Answer from the drawing. Dimensions are ordinates in mm from the lowest x, y and z of the part. A direction names the side the tool comes from. Round coordinates to 2 decimals unless told otherwise and drop trailing zeros. Loops run counter-clockwise (first coordinate to the right, second up) from the corner with the lowest first, then second, coordinate; pieces in that order, holes last. Notation, with made-up numbers: M -29.5,42.25 L -22.5,42.25 A26 cw -22.5,69.25 Z; hole C -15,2 d6. An arc over 180 degrees is marked long. One line per item, written item: value.
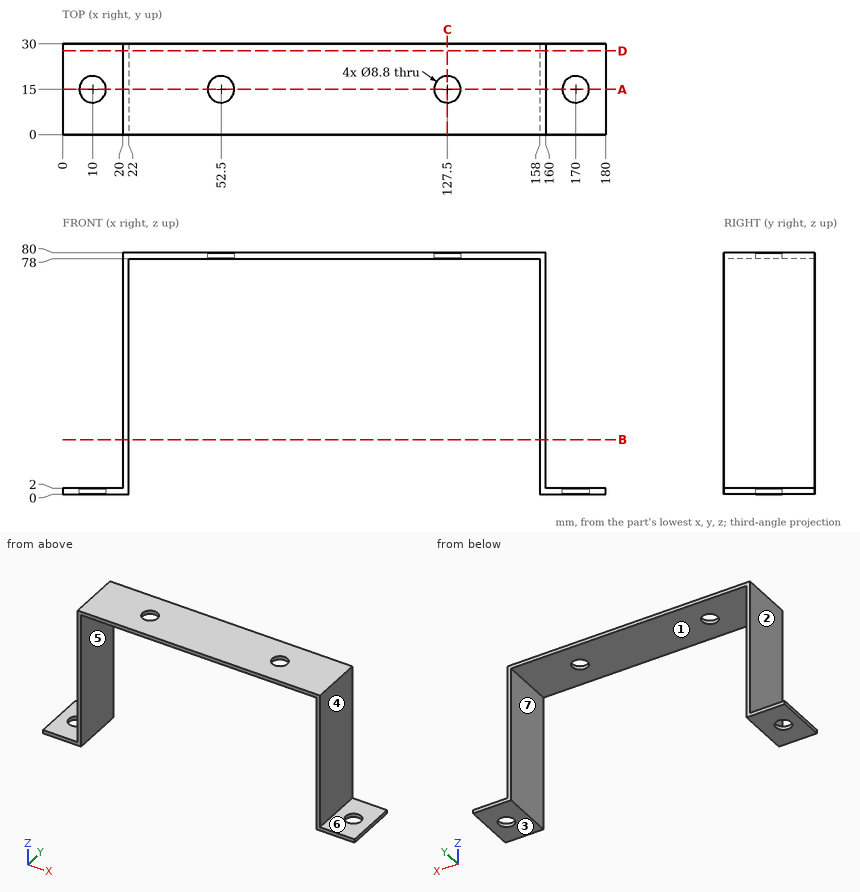
1) The mould has two halves that part along X. Classify the marked faces 4, 5, 6 and 7: +X half, -X half, draft (parallel to the pull), parting line (faces both ways), or undercut.
Check values:
face 4: +X half
face 5: undercut
face 6: draft
face 7: undercut
2) Find the intervals of material crossed by probe 1 along X at (y, z) = (10.5, 19); probe 2 along Y at (x, z) = (127.5, 79.1); probe 3 along Z at (x, y) = (111.5, 21.25), in increasing order. Write a range as from..to.
Check values:
probe 1: 20..22, 158..160
probe 2: 0..10.6, 19.4..30
probe 3: 78..80
3) Find section A-A (y = 15). Give the vertices of the cut face in (x, z).
Check values:
outline: M 0,0 L 5.6,0 L 5.6,2 L 0,2 Z; M 14.4,0 L 22,0 L 22,78 L 48.1,78 L 48.1,80 L 20,80 L 20,2 L 14.4,2 Z; M 56.9,78 L 123.1,78 L 123.1,80 L 56.9,80 Z; M 131.9,78 L 158,78 L 158,0 L 165.6,0 L 165.6,2 L 160,2 L 160,80 L 131.9,80 Z; M 174.4,0 L 180,0 L 180,2 L 174.4,2 Z
4) For the marked faces 1, 2 and 3, determine the directions among +Z, -Z, +X, -X, +Y, -Y from which every point of the face is accessible in a straight line to the end or side of a thin tool.
Check values:
face 1: -Z, +Y, -Y
face 2: +Z, -X, +Y, -Y
face 3: -Z, +X, -X, +Y, -Y
5) Find section D-D (y = 27.75). Give the vertices of the cut face in (x, z), then the cut area to 3 significant figures.
Check values:
outline: M 0,0 L 22,0 L 22,78 L 158,78 L 158,0 L 180,0 L 180,2 L 160,2 L 160,80 L 20,80 L 20,2 L 0,2 Z
area: 672 mm2
6) Each of these flat-tipped pins is pushed along its axis until it touches: pin 1 (8 mm diameter, centred on y = 12.5, z = 28, fed in from -X); pin 2 (10 mm diameter, centred on x = 170, y = 15, fed in from +Z); pin 3 (3 mm diameter, centred on y = 23, z = 35.5, fed in from +X). Where does it stop, or does it pass through?
Check values:
pin 1: x = 20
pin 2: z = 2
pin 3: x = 160
7) Find section C-C (x = 127.5). Give the vertices of the cut face in (y, z), then the cut area to 3 significant figures.
Check values:
outline: M 0,78 L 10.6,78 L 10.6,80 L 0,80 Z; M 19.4,78 L 30,78 L 30,80 L 19.4,80 Z
area: 42.4 mm2
8) Find section B-B (z = 18). Give the vertices of the cut face in (x, y).
Check values:
outline: M 20,0 L 22,0 L 22,30 L 20,30 Z; M 158,0 L 160,0 L 160,30 L 158,30 Z
